Here's how the part is built. I have some questions about the finished solid (model axes, mm). A direction names the side the tool comes from. Give positions to 0.01 mm unless a question says otherwise; leave off trailing zeros. Loops run counter-clockwise (first coordinate to the right, second up) from the corner with the lowest first, then second, coordinate; pieces in that order, holes last. Notation, with made-up numbers: (30.25, 51) - (77.25, 51) arc R18 cw to (77.25, 59) - close; hole circle Ø7 at (7.5, 0). An arc over 180 degrees is marked (long way). Return JSON: item names as keys, results as strings. Group by question number.
(1) For P1, Ø1.7, axis at x = -2, z = -1.5, coming from the -Y side; P2, Ø1, axis at x = -1, y = 1.5, coming from the -Z side, each with a flat end and sliding along its axis, tell me the tip position at first contact or that it passes through.
(2) I need wall thicknesses on probe 1 along X at (y, z) = (1.5, 3) (1 decimal); probe 2 along Y at (x, z) = (4.25, -1.5); probe 3 along X at (y, z) = (0.6, 0). Which ranges of each line are inside material? Lowest first, please. Write a range as [from, to].
(3) If we section it at C-C (x = 6): Please give me the cut outline in (y, z).
(4) If we section it at B-B (y = 2.7): Please give me the cut outline in (x, z), then the cut area to 3 significant figures.
(5) On a 3-axis mill with a long thin cutter (end or side, diameter ignored), from which of +Z, -Z, +X, -X, +Y, -Y can I reach the whole of each face in a straight line? I mean faces 4 (the flat face through (7.401, 3.157, 5.567)), 5 (the flat face through (11, 1.588, 0)), 6 (the flat face through (-2, 0.794, 0)), 7 (the flat face through (1.588, 1, 0)). Say none if no direction works.
(6) If we mould it in two halves opening along Z, with no side actions, what happens to faces 1 (the flat face through (14.288, 1, 0)), 2 (the flat face through (6, 2, 6.35)), 3 (the flat face through (7, 3, -4.762))? For each: released by +Z, released by -Z, zero draft, split by the parting line, or undercut.
```python
from build123d import *

# Parameters (mm, degrees)
BOSS_EXTRUDE1_DEPTH            = 6.35
CUT_EXTRUDE3_START             = 1.5875
SKETCH4_W                      = 11.1125
SKETCH4_H                      = 9.525
CUT_EXTRUDE3_DEPTH             = 4.175
CUT_EXTRUDE4_REACH             = 8.35
CUT_EXTRUDE4_DIRECTION_2_REACH = 8.35
SKETCH3_R                      = 2.579687
CUT_EXTRUDE2_DEPTH             = 2.54


with BuildPart() as part:
    # Sketch1 → Boss-Extrude1 (new body, symmetric)
    with BuildSketch(Plane.XY):
        with BuildLine():
            Line((-3.175, 0.79375), (-3.175, 1.5875))
            ThreePointArc((-3.175, 1.5875), (-1.97996, 4.069512), (0.705556, 4.683112))
            Line((0.705556, 4.683112), (14.2875, 1.5875))
            Line((14.2875, 1.5875), (14.2875, 0))
            Line((14.2875, 0), (1.5875, 0))
            Line((1.5875, 0), (1.5875, 1.5875))
            ThreePointArc((1.5875, 1.5875), (0, 3.175), (-1.5875, 1.5875))
            Line((-1.5875, 1.5875), (-1.5875, 0.79375))
            Line((-1.5875, 0.79375), (-3.175, 0.79375))
        make_face()
    extrude(amount=BOSS_EXTRUDE1_DEPTH, both=True)

    # Sketch4 → Cut-Extrude3 (cut, through all)
    with BuildSketch(Plane(origin=(0, 0, 0), x_dir=(1, 0, 0), z_dir=(0, 1, 0)).offset(CUT_EXTRUDE3_START)):
        with Locations((8.73125, 0)):
            Rectangle(SKETCH4_W, SKETCH4_H)
    extrude(amount=CUT_EXTRUDE3_DEPTH, mode=Mode.SUBTRACT)

    # Cut-Extrude4: up to this face of the body (flat: up to its plane)
    cut_extrude4_end = Plane(part.part.faces().sort_by_distance((6.879167, 2.431758, 4.7625))[0])
    # Sketch5 → Cut-Extrude4 (cut, up to the picked face)
    with BuildSketch(Plane.XY, mode=Mode.PRIVATE) as cut_extrude4_sk1:
        with BuildLine():
            Line((3.175, 1.5875), (3.175, 4.120274))
            Line((3.175, 4.120274), (0.705556, 4.683112))
            ThreePointArc((0.705556, 4.683112), (2.482012, 3.56746), (3.175, 1.5875))
        make_face()
    cut_extrude4_tool1 = split(extrude(cut_extrude4_sk1.sketch, amount=CUT_EXTRUDE4_REACH, mode=Mode.PRIVATE), bisect_by=cut_extrude4_end, keep=Keep.BOTH, mode=Mode.PRIVATE)
    add(cut_extrude4_tool1.solids().sort_by_distance((2.639834, 3.693359, 0))[0], mode=Mode.SUBTRACT)

    # Cut-Extrude4 direction 2: up to this face of the body (flat: up to its plane)
    cut_extrude4_direction_2_end = Plane(part.part.faces().sort_by_distance((6.879167, 2.431758, -4.7625))[0])
    # Sketch5 → Cut-Extrude4 direction 2 (cut, up to the picked face)
    with BuildSketch(Plane.XY, mode=Mode.PRIVATE) as cut_extrude4_direction_2_sk1:
        with BuildLine():
            Line((3.175, 1.5875), (3.175, 4.120274))
            Line((3.175, 4.120274), (0.705556, 4.683112))
            ThreePointArc((0.705556, 4.683112), (2.482012, 3.56746), (3.175, 1.5875))
        make_face()
    cut_extrude4_direction_2_tool1 = split(extrude(cut_extrude4_direction_2_sk1.sketch, amount=-CUT_EXTRUDE4_DIRECTION_2_REACH, mode=Mode.PRIVATE), bisect_by=cut_extrude4_direction_2_end, keep=Keep.BOTH, mode=Mode.PRIVATE)
    add(cut_extrude4_direction_2_tool1.solids().sort_by_distance((2.639834, 3.693359, 0))[0], mode=Mode.SUBTRACT)

    # Sketch3 → Cut-Extrude2 (cut)
    with BuildSketch(Plane(origin=(0, 0, 0), x_dir=(1, 0, 0), z_dir=(0, 1, 0))):
        with Locations((7.9375, 0)):
            Circle(SKETCH3_R)
    extrude(amount=CUT_EXTRUDE2_DEPTH, mode=Mode.SUBTRACT)


solid = part.part
```
Values:
{
 "1": {"P1": "y = 0.79", "P2": "through"},
 "2": {"probe 1": "[-3.2, -1.6], [1.6, 14.3]", "probe 2": "[0, 1.59]", "probe 3": "[1.59, 5.36], [10.52, 14.29]"},
 "3": {"outline": "(0, -6.35) - (3.48, -6.35) - (3.48, -4.76) - (1.59, -4.76) - (1.59, -1.7) - (0, -1.7) - close; (0, 1.7) - (1.59, 1.7) - (1.59, 4.76) - (3.48, 4.76) - (3.48, 6.35) - (0, 6.35) - close"},
 "4": {"outline": "(-2.97, -6.35) - (-1.13, -6.35) - (-1.13, 6.35) - (-2.97, 6.35) - close; (1.13, -6.35) - (9.41, -6.35) - (9.41, -4.76) - (2.97, -4.76) - (2.97, 4.76) - (9.41, 4.76) - (9.41, 6.35) - (1.13, 6.35) - close", "area": "67.2 mm2"},
 "5": {"face 4": "+Z, -Z, +X, +Y", "face 5": "+X, +Y", "face 6": "+Z, -Z, -X, -Y", "face 7": "+Z, -Z, -Y"},
 "6": {"face 1": "zero draft", "face 2": "released by +Z", "face 3": "undercut"}
}
